Design review of the part built by this model. Coordinates are the model's own, in mm. A direction names the side the tool comes from. Coordinates: 2 decimals unless noted, no trailing zeros. Loops run counter-clockwise (first coordinate to the right, second up) from the corner with the lowest first, then second, coordinate; pieces in that order, holes last. Notation, with made-up numbers: (79.5, 13.25) - (99.5, 13.25) arc R19 ccw to (99.5, 22.25) - close; hole circle Ø11 at (-36.5, -37.75). An arc over 180 degrees is marked (long way). Use one line per item in the form item = value. Start each with the question number.
(1) The part is to be moulded in two halves that separate along X. For faces 1 (the face through (5, 10, 0)), 2 (the face through (-1.73, 4.24, -7.81)), 3 (the face through (17.13, 2.38, -20.85)), say which applies: pulls with the +X half, pulls with the -X half, needs draft (parallel to the pull), parting line crosses it, or undercut.
(2) Add section B-B (z = 0). State the section outline as (x, y) points, plus the area to 3 significant figures.
(3) Tool access review of faces 4 (the face through (-9.4, 8, -14)), 5 (the face through (18.057, -1.282, -18.147)), 6 (the face through (17.13, 2.52, 20.85)): name each direction out of +Z, -Z, +X, -X, +Y, -Y from which nothing blocks a thin tool from reaching the whole face with its end or side.
(4) Add section D-D (y = 6.5). State the section outline as (x, z) points.
(5) Clearance check with flat-ended pins moving along their axes: pin 1 Ø4 at (x, z) = (15.5, 15.5) entering from -Y; pin 2 Ø13 at (x, z) = (0, 0.5) entering from -Y; pin 3 Ø6.5 at (x, z) = (0, 0) entering from +Y; pin 4 Ø4 at (x, z) = (-15.5, -15.5) entering from +Y. State where each tip first meets the part, or that it passes through.
(6) For L1, parallel to X at y = 4.5, z = -15.5; L2, parallel to X at y = 8.9, z = 0, list the stretches that pass through material, from the lowest coordinate up.
(7) Add section C-C (y = -1.5). State the section outline as (x, z) points.
(8) Add section A-A (x = 0). State the section outline as (y, z) points.
```python
from build123d import *

# Parameters (mm, degrees)
SKETCH_1_R          = 2.65
SKETCH_1_R_2        = 16.5
SKETCH_1_R_3        = 1.25
EXTRUDE_1_DEPTH     = 8
SKETCH_1_3_R        = 16.5
SKETCH_1_3_R_2      = 11
EXTRUDE_2_DEPTH     = 7.5
SKETCH_1_4_R        = 11
SKETCH_1_4_R_2      = 3.65
EXTRUDE_3_DEPTH     = 10
EXTRUDE_4_DEPTH     = 2.6
SKETCH_2_R          = 8
CUT_EXTRUDE_1_DEPTH = 8.6
FILLET_1_R          = 2
FILLET_2_R          = 0.5
CHAMFER_1_SIZE      = 0.3


with BuildPart() as part:
    # Sketch 1 → Extrude 1 (new body)
    with BuildSketch(Plane(origin=(0, 0, 0), x_dir=(1, 0, 0), z_dir=(0, 1, 0))):
        with BuildLine():
            ThreePointArc((-14.641038215, 21), (-18.101933598, 18.101933598), (-21, 14.641038215))
            Line((-21, 14.641038215), (-21, -14.641038215))
            ThreePointArc((-21, -14.641038215), (-18.101933598, -18.101933598), (-14.641038215, -21))
            Line((-14.641038215, -21), (14.641038215, -21))
            ThreePointArc((14.641038215, -21), (18.101933598, -18.101933598), (21, -14.641038215))
            Line((21, -14.641038215), (21, 14.641038215))
            ThreePointArc((21, 14.641038215), (18.101933598, 18.101933598), (14.641038215, 21))
            Line((14.641038215, 21), (-14.641038215, 21))
        make_face()
        with Locations((-15.5, -15.5)):
            Circle(SKETCH_1_R, mode=Mode.SUBTRACT)
        with Locations((15.5, -15.5)):
            Circle(SKETCH_1_R, mode=Mode.SUBTRACT)
        Circle(SKETCH_1_R_2, mode=Mode.SUBTRACT)
        with Locations((-15.5, 15.5)):
            Circle(SKETCH_1_R, mode=Mode.SUBTRACT)
        with Locations((15.5, 15.5)):
            Circle(SKETCH_1_R, mode=Mode.SUBTRACT)
        with Locations((15.5, -15.5)):
            Circle(SKETCH_1_R)
        with Locations((15.5, -15.5)):
            Circle(SKETCH_1_R_3, mode=Mode.SUBTRACT)
        with Locations((-15.5, -15.5)):
            Circle(SKETCH_1_R)
        with Locations((-15.5, -15.5)):
            Circle(SKETCH_1_R_3, mode=Mode.SUBTRACT)
        with Locations((-15.5, 15.5)):
            Circle(SKETCH_1_R)
        with Locations((-15.5, 15.5)):
            Circle(SKETCH_1_R_3, mode=Mode.SUBTRACT)
        with Locations((15.5, 15.5)):
            Circle(SKETCH_1_R)
        with Locations((15.5, 15.5)):
            Circle(SKETCH_1_R_3, mode=Mode.SUBTRACT)
        with BuildLine():
            ThreePointArc((-14.641038215, -21), (-18.101933598, -18.101933598), (-21, -14.641038215))
            Line((-21, -14.641038215), (-21, -17.2))
            Line((-21, -17.2), (-17.2, -21))
            Line((-17.2, -21), (-14.641038215, -21))
        make_face()
        with BuildLine():
            Line((-17.2, 21), (-21, 17.2))
            Line((-21, 17.2), (-21, 14.641038215))
            ThreePointArc((-21, 14.641038215), (-18.101933598, 18.101933598), (-14.641038215, 21))
            Line((-14.641038215, 21), (-17.2, 21))
        make_face()
        with BuildLine():
            Line((17.2, 21), (14.641038215, 21))
            ThreePointArc((14.641038215, 21), (18.101933598, 18.101933598), (21, 14.641038215))
            Line((21, 14.641038215), (21, 17.2))
            Line((21, 17.2), (17.2, 21))
        make_face()
        with BuildLine():
            ThreePointArc((21, -14.641038215), (18.101933598, -18.101933598), (14.641038215, -21))
            Line((14.641038215, -21), (17.2, -21))
            Line((17.2, -21), (21, -17.2))
            Line((21, -17.2), (21, -14.641038215))
        make_face()
    extrude(amount=EXTRUDE_1_DEPTH)

    # Sketch 1_3 → Extrude 2 (add)
    with BuildSketch(Plane(origin=(0, 0, 0), x_dir=(1, 0, 0), z_dir=(0, 1, 0))):
        Circle(SKETCH_1_3_R)
        Circle(SKETCH_1_3_R_2, mode=Mode.SUBTRACT)
    extrude(amount=EXTRUDE_2_DEPTH)

    # Sketch 1_4 → Extrude 3 (add)
    with BuildSketch(Plane(origin=(0, 0, 0), x_dir=(1, 0, 0), z_dir=(0, 1, 0))):
        Circle(SKETCH_1_4_R)
        Circle(SKETCH_1_4_R_2, mode=Mode.SUBTRACT)
    extrude(amount=EXTRUDE_3_DEPTH)

    # Sketch 1_5 → Extrude 4 (add)
    with BuildSketch(Plane(origin=(0, 0, 0), x_dir=(1, 0, 0), z_dir=(0, 1, 0))):
        with BuildLine():
            ThreePointArc((-14.641038215, -21), (-18.101933598, -18.101933598), (-21, -14.641038215))
            Line((-21, -14.641038215), (-21, -17.2))
            Line((-21, -17.2), (-17.2, -21))
            Line((-17.2, -21), (-14.641038215, -21))
        make_face()
        with BuildLine():
            ThreePointArc((21, -14.641038215), (18.101933598, -18.101933598), (14.641038215, -21))
            Line((14.641038215, -21), (17.2, -21))
            Line((17.2, -21), (21, -17.2))
            Line((21, -17.2), (21, -14.641038215))
        make_face()
        with BuildLine():
            Line((-17.2, 21), (-21, 17.2))
            Line((-21, 17.2), (-21, 14.641038215))
            ThreePointArc((-21, 14.641038215), (-18.101933598, 18.101933598), (-14.641038215, 21))
            Line((-14.641038215, 21), (-17.2, 21))
        make_face()
        with BuildLine():
            Line((17.2, 21), (14.641038215, 21))
            ThreePointArc((14.641038215, 21), (18.101933598, 18.101933598), (21, 14.641038215))
            Line((21, 14.641038215), (21, 17.2))
            Line((21, 17.2), (17.2, 21))
        make_face()
    extrude(amount=-EXTRUDE_4_DEPTH)

    # Sketch 2 → Cut-Extrude 1 (cut)
    with BuildSketch(Plane.XZ):
        Circle(SKETCH_2_R)
    extrude(amount=-CUT_EXTRUDE_1_DEPTH, mode=Mode.SUBTRACT)

    # Fillet 1
    fillet_1_edges = [part.edges().sort_by_distance(p)[0] for p in [
        (-17.2, 2.7, 21),
        (-21, 2.7, 17.2),
        (-21, 2.7, -17.2),
        (-17.2, 2.7, -21),
        (17.2, 2.7, -21),
        (21, 2.7, -17.2),
        (21, 2.7, 17.2),
        (17.2, 2.7, 21),
    ]]
    fillet(fillet_1_edges, radius=FILLET_1_R)

    # Fillet 2
    fillet_2_edges = [part.edges().sort_by_distance(p)[0] for p in [
        (21, 8, 0),
        (19.1, 8, 19.1),
        (0, 8, 21),
        (19.1, 8, -19.1),
        (0, 8, -21),
        (-19.1, 8, -19.1),
        (-21, 8, 0),
        (-19.1, 8, 19.1),
        (20.847759065, 8, -17.13693974),
        (17.13693974, 8, -20.847759065),
        (-17.13693974, 8, -20.847759065),
        (-20.847759065, 8, -17.13693974),
        (-20.847759065, 8, 17.13693974),
        (-17.13693974, 8, 20.847759065),
        (17.13693974, 8, 20.847759065),
        (20.847759065, 8, 17.13693974),
        (-3.65, 10, 0),
        (-11, 10, 0),
    ]]
    fillet(fillet_2_edges, radius=FILLET_2_R)

    # Chamfer 1
    chamfer_1_edges = [part.edges().sort_by_distance(p)[0] for p in [
        (-16.75, 8, -15.5),
        (14.25, 8, -15.5),
        (14.25, 8, 15.5),
        (-16.75, 8, 15.5),
    ]]
    chamfer(chamfer_1_edges, length=CHAMFER_1_SIZE)


solid = part.part
```
Computed values:
q1.face_1 = needs draft
q1.face_2 = undercut
q1.face_3 = pulls with the +X half
q2.outline = (-21, 0) - (-8, 0) - (-8, 8.6) - (-3.65, 8.6) - (-3.65, 9.5) arc R0.5 ccw to (-4.15, 10) - (-10.5, 10) arc R0.5 ccw to (-11, 9.5) - (-11, 7.5) - (-16.5, 7.5) - (-16.5, 8) - (-20.5, 8) arc R0.5 ccw to (-21, 7.5) - close; (3.65, 8.6) - (8, 8.6) - (8, 0) - (21, 0) - (21, 7.5) arc R0.5 ccw to (20.5, 8) - (16.5, 8) - (16.5, 7.5) - (11, 7.5) - (11, 9.5) arc R0.5 ccw to (10.5, 10) - (4.15, 10) arc R0.5 ccw to (3.65, 9.5) - close
q2.area = 226 mm^2
q3.face_4 = +Y
q3.face_5 = -Y
q3.face_6 = +Z, +X, +Y, -Y
q4.outline = (-21, -16.37) arc R2 ccw to (-20.41, -17.79) - (-17.79, -20.41) arc R2 ccw to (-16.37, -21) - (16.37, -21) arc R2 ccw to (17.79, -20.41) - (20.41, -17.79) arc R2 ccw to (21, -16.37) - (21, 16.37) arc R2 ccw to (20.41, 17.79) - (17.79, 20.41) arc R2 ccw to (16.37, 21) - (-16.37, 21) arc R2 ccw to (-17.79, 20.41) - (-20.41, 17.79) arc R2 ccw to (-21, 16.37) - close; hole circle Ø2.5 at (-15.5, -15.5); hole circle Ø2.5 at (-15.5, 15.5); hole circle Ø16 at (0, 0); hole circle Ø2.5 at (15.5, -15.5); hole circle Ø2.5 at (15.5, 15.5)
q5.pin_1 = 0
q5.pin_2 = 8.6
q5.pin_3 = through
q5.pin_4 = 8
q6.L1 = -21 to -16.75, -14.25 to 14.25, 16.75 to 21
q6.L2 = -11 to -3.65, 3.65 to 11
q7.outline = (-21, -16.37) arc R2 ccw to (-20.41, -17.79) - (-17.79, -20.41) arc R2 ccw to (-16.37, -21) - (-14.64, -21) arc R25.6 cw to (-21, -14.64) - close; (-21, 14.64) arc R25.6 cw to (-14.64, 21) - (-16.37, 21) arc R2 ccw to (-17.79, 20.41) - (-20.41, 17.79) arc R2 ccw to (-21, 16.37) - close; (14.64, -21) - (16.37, -21) arc R2 ccw to (17.79, -20.41) - (20.41, -17.79) arc R2 ccw to (21, -16.37) - (21, -14.64) arc R25.6 cw to start; (14.64, 21) arc R25.6 cw to (21, 14.64) - (21, 16.37) arc R2 ccw to (20.41, 17.79) - (17.79, 20.41) arc R2 ccw to (16.37, 21) - close
q8.outline = (0, -21) - (7.5, -21) arc R0.5 ccw to (8, -20.5) - (8, -16.5) - (7.5, -16.5) - (7.5, -11) - (9.5, -11) arc R0.5 ccw to (10, -10.5) - (10, -4.15) arc R0.5 ccw to (9.5, -3.65) - (8.6, -3.65) - (8.6, -8) - (0, -8) - close; (0, 8) - (8.6, 8) - (8.6, 3.65) - (9.5, 3.65) arc R0.5 ccw to (10, 4.15) - (10, 10.5) arc R0.5 ccw to (9.5, 11) - (7.5, 11) - (7.5, 16.5) - (8, 16.5) - (8, 20.5) arc R0.5 ccw to (7.5, 21) - (0, 21) - close
